Check sheet for the modelled part. Datum: model origin and axes. Units: mm. A direction names the side the tool comes from. Round coordinates to 2 decimals unless told otherwise and drop trailing zeros. Loops run counter-clockwise (first coordinate to the right, second up) from the corner with the lowest first, then second, coordinate; pieces in that order, holes last. Notation, with made-up numbers: (-38.5, 73.25) -> (-32.5, 73.25) arc R19 ccw to (-32.5, 104.25) -> close; hole circle Ø8 at (72, 80). An arc over 180 degrees is marked (long way). One line per question, with ' | ' between items.
```python
from build123d import *

# Parameters (mm, degrees)
F0_W     = 50.8
F0_H     = 66.04
F1_DEPTH = 5.08
F0_H_2   = 5.08
F2_DEPTH = 38.1


with BuildPart() as f1:
    # F0 (on Top) → F1 (new body)
    with BuildSketch(Plane.XY):
        with BuildLine():
            ThreePointArc((0, -31.75), (-31.75, 0), (0, 31.75))
            Line((0, 31.75), (0, 97.79))
            ThreePointArc((0, 97.79), (-97.79, 0), (0, -97.79))
            Line((0, -97.79), (0, -31.75))
        make_face()
        with Locations((25.4, -64.77)):
            Rectangle(F0_W, F0_H)
        with Locations((25.4, 64.77)):
            Rectangle(F0_W, F0_H)
    extrude(amount=F1_DEPTH)

    # F0 (on Top) → F2 (join)
    with BuildSketch(Plane.XY):
        with BuildLine():
            ThreePointArc((0, -97.79), (-97.79, 0), (0, 97.79))
            Line((0, 97.79), (0, 102.87))
            ThreePointArc((0, 102.87), (-102.87, 0), (0, -102.87))
            Line((0, -102.87), (0, -97.79))
        make_face()
        with Locations((25.4, -100.33)):
            Rectangle(F0_W, F0_H_2)
        with BuildLine():
            Line((0, 26.67), (0, 31.75))
            ThreePointArc((0, 31.75), (-31.75, 0), (0, -31.75))
            Line((0, -31.75), (0, -26.67))
            ThreePointArc((0, -26.67), (-26.67, 0), (0, 26.67))
        make_face()
        with Locations((25.4, -29.21)):
            Rectangle(F0_W, F0_H_2)
        with Locations((25.4, 29.21)):
            Rectangle(F0_W, F0_H_2)
        with Locations((25.4, 100.33)):
            Rectangle(F0_W, F0_H_2)
    extrude(amount=F2_DEPTH)


solid = f1.part
```
(1) Sectioned sample at B-B, the plane x = -15.5. Record the cut outline in (y, z).
Answer:
outline: (-101.7, 0) -> (-21.7, 0) -> (-21.7, 38.1) -> (-27.71, 38.1) -> (-27.71, 5.08) -> (-96.55, 5.08) -> (-96.55, 38.1) -> (-101.7, 38.1) -> close; (21.7, 0) -> (101.7, 0) -> (101.7, 38.1) -> (96.55, 38.1) -> (96.55, 5.08) -> (27.71, 5.08) -> (27.71, 38.1) -> (21.7, 38.1) -> close
(2) Set-up check for faces 1 (the face through (25, 97.79, 21)), 2 (the face through (50.8, 64.6, 4.8)), 3 (the face through (-41, 1, 5.08)), 4 (the face through (25, -26.67, 19)): record each of +Z, -Z, +X, -X, +Y, -Y from which the full face is reachable in a straight line by a thin tool's end or side.
Answer:
face 1: +Z, +X | face 2: +Z, -Z, +X, +Y, -Y | face 3: +Z | face 4: +Z, -Z, +X
(3) Scan lines: probe 1 along Y at (x, z) = (28, 17); probe 2 along Z at (x, y) = (-59, 61.5). Record each from-to range of solid material in increasing order.
Answer:
probe 1: y = -102.87 to -97.79, -31.75 to -26.67, 26.67 to 31.75, 97.79 to 102.87 | probe 2: z = 0 to 5.08
(4) Sectioned sample at C-C, the plane y = 0. Record the cut outline in (x, z).
Answer:
outline: (-102.87, 0) -> (-26.67, 0) -> (-26.67, 38.1) -> (-31.75, 38.1) -> (-31.75, 5.08) -> (-97.79, 5.08) -> (-97.79, 38.1) -> (-102.87, 38.1) -> close
(5) Go/stop test with flat-tipped pins: pin 1 (6 mm diameter, centred on x = -29, y = -44, fed in from +Z); pin 2 (10 mm diameter, centred on y = -12.5, z = 32, fed in from -X); pin 3 (3 mm diameter, centred on x = -53.5, z = 18.5, fed in from +Y). Record where each tip stops, or that it passes through.
Answer:
pin 1: stops at z = 5.08 | pin 2: stops at x = -102.6 | pin 3: stops at y = 88.76
(6) Sectioned sample at A-A, the plane z = 22. Record the cut outline in (x, y).
Answer:
outline: (0, -102.87) -> (50.8, -102.87) -> (50.8, -97.79) -> (0, -97.79) arc R97.79 cw to (0, 97.79) -> (50.8, 97.79) -> (50.8, 102.87) -> (0, 102.87) arc R102.87 ccw to start; (0, -31.75) -> (50.8, -31.75) -> (50.8, -26.67) -> (0, -26.67) arc R26.67 cw to (0, 26.67) -> (50.8, 26.67) -> (50.8, 31.75) -> (0, 31.75) arc R31.75 ccw to start
(7) Mould release check, pull along Y, two halves, no side actions. Record for faces 5 (the face through (-100, 0, 38.1)), 6 (the face through (-31.742, 0.698, 21.359)), 7 (the face through (25, -102.87, 19)): +Y half, -Y half, draft (parallel to the pull), parting line (faces both ways), or undercut.
Answer:
face 5: draft | face 6: undercut | face 7: -Y half
(8) Sectioned sample at D-D, the plane x = -77.5. Record the cut outline in (y, z), and give its area (3 significant figures).
Answer:
outline: (-67.65, 0) -> (67.65, 0) -> (67.65, 38.1) -> (59.64, 38.1) -> (59.64, 5.08) -> (-59.64, 5.08) -> (-59.64, 38.1) -> (-67.65, 38.1) -> close | area: 1,220 mm2
